```python
from build123d import *

# Parameters (mm, degrees)
SKETCH2_R              = 14.2875
SKETCH2_W              = 81.28
SKETCH2_H              = 3.175
BOSS_EXTRUDE1_DEPTH    = 3.175
SKETCH9_R              = 14.2875
CUT_EXTRUDE2_DEPTH     = 3.175
SKETCH2_3_W            = 81.28
SKETCH2_3_H            = 3.175
BOSS_EXTRUDE2_DEPTH    = 60.7695
BOSS_EXTRUDE3_DEPTH    = 3.175
FILLET1_R              = 2.54
FILLET2_R              = 42.2275
CONVERT_SOLID2_START   = -102
CONVERT_SOLID2_DEPTH   = 184
CONVERT_SOLID2_2_DEPTH = 81.28
UNFOLD1_START          = -51
UNFOLD1_DEPTH          = 132.28
UNFOLD1_2_DEPTH        = 78.74
UNFOLD1_START_2        = 0.13716
UNFOLD1_3_DEPTH        = 3.03784
FOLD1_START            = -58.892012294
FOLD1_OUTLINE_W        = 3.03784
FOLD1_OUTLINE_H        = 81.28
FOLD1_DEPTH            = 59.530319476
FOLD1_2_DEPTH          = 6.21284
FOLD1_START_2          = -49.557397552
FOLD1_3_DEPTH          = 131.557397552


with BuildPart() as part:
    # Sketch2 → Boss-Extrude1 (new body)
    # profile 1 of 2: a face of its own
    with BuildSketch(Plane(origin=(0, 0, 0), x_dir=(0, 0, -1), z_dir=(1, 0, 0))):
        with BuildLine():
            Line((0, 3.175), (0, 69.85))
            Line((0, 69.85), (89.183866464, 160.063269699))
            ThreePointArc((89.183866464, 160.063269699), (97.582743975, 203.257963311), (60.96, 227.65258))
            Line((60.96, 227.65258), (-81.28, 227.65258))
            Line((-81.28, 227.65258), (-81.28, 69.85))
            Line((-81.28, 69.85), (-81.28, 3.175))
            Line((-81.28, 3.175), (0, 3.175))
        make_face()
        with Locations((60.96, 187.96508)):
            Circle(SKETCH2_R, mode=Mode.SUBTRACT)
    # profile 2 of 2: a face of its own
    with BuildSketch(Plane(origin=(0, 0, 0), x_dir=(0, 0, -1), z_dir=(1, 0, 0))):
        with Locations((-40.64, 1.5875)):
            Rectangle(SKETCH2_W, SKETCH2_H)
    extrude(amount=BOSS_EXTRUDE1_DEPTH)

    # Sketch9 → Cut-Extrude2 (cut)
    with BuildSketch(Plane(origin=(0, 0, 0), x_dir=(0, 0, -1), z_dir=(1, 0, 0))):
        with Locations((-49.5046, 74.46228868)):
            Circle(SKETCH9_R)
    extrude(amount=CUT_EXTRUDE2_DEPTH, mode=Mode.SUBTRACT)

    # Sketch2<3> → Boss-Extrude2 (add)
    with BuildSketch(Plane(origin=(0, 0, 0), x_dir=(0, 0, -1), z_dir=(1, 0, 0))):
        with Locations((-40.64, 1.5875)):
            Rectangle(SKETCH2_3_W, SKETCH2_3_H)
    extrude(amount=-BOSS_EXTRUDE2_DEPTH)

    # Sketch3 → Boss-Extrude3 (add)
    with BuildSketch(Plane(origin=(0, 3.175, 0), x_dir=(1, 0, 0), z_dir=(0, 1, 0))):
        Polygon((-60.7695, 0), (-60.7695, 53.1495), (-7.62, 0), align=None)
    extrude(amount=-BOSS_EXTRUDE3_DEPTH)

    # Fillet1
    fillet1_edges = [part.edges().sort_by_distance(p)[0] for p in [
        (-60.7695, 1.5875, 81.28),
        (-60.7695, 1.5875, -53.1495),
    ]]
    fillet(fillet1_edges, radius=FILLET1_R)

    # Fillet2
    fillet2_edges = [part.edges().sort_by_distance(p)[0] for p in [
        (1.5875, 227.65258, 81.28),
    ]]
    fillet(fillet2_edges, radius=FILLET2_R)

    # Convert-Solid2: read off the stored shape, not the designer's step
    # Convert-Solid2 outline → Convert-Solid2 (cut)
    with BuildSketch(Plane.XY.offset(CONVERT_SOLID2_START)):
        with BuildLine():
            ThreePointArc((3.175, 6.21284), (1.355301294, 1.819698706), (-3.03784, 0))
            Line((-3.03784, 0), (3.175, 0))
            Line((3.175, 0), (3.175, 6.21284))
        make_face()
        with BuildLine():
            Line((-60.7695, 3.175), (-60.7695, 3.03784))
            Line((-60.7695, 3.03784), (-3.03784, 3.03784))
            ThreePointArc((-3.03784, 3.03784), (-2.571212204, 3.072317193), (-2.114718593, 3.175))
            Line((-2.114718593, 3.175), (-60.7695, 3.175))
        make_face()
        with BuildLine():
            Line((0.13716, 6.21284), (0.13716, 227.65258))
            Line((0.13716, 227.65258), (0, 227.65258))
            Line((0, 227.65258), (0, 5.289718593))
            ThreePointArc((0, 5.289718593), (0.102682807, 5.746212204), (0.13716, 6.21284))
        make_face()
    extrude(amount=CONVERT_SOLID2_DEPTH, mode=Mode.SUBTRACT)

    # Convert-Solid2 2 outline → Convert-Solid2 2 (add)
    with BuildSketch(Plane.XY):
        with BuildLine():
            ThreePointArc((0, 5.289718593), (-0.79277597, 3.96777597), (-2.114718593, 3.175))
            Line((-2.114718593, 3.175), (0, 3.175))
            Line((0, 3.175), (0, 5.289718593))
        make_face()
    extrude(amount=CONVERT_SOLID2_2_DEPTH)

    # Unfold1: read off the stored shape, not the designer's step
    # Unfold1 outline → Unfold1 (cut)
    with BuildSketch(Plane.XY.offset(UNFOLD1_START)):
        with BuildLine():
            ThreePointArc((-3.03784, 0), (-1.391483498, 0.222106228), (0.13716, 0.872544516))
            Line((0.13716, 0.872544516), (0.13716, 6.21284))
            ThreePointArc((0.13716, 6.21284), (-0.79277597, 3.96777597), (-3.03784, 3.03784))
            Line((-3.03784, 3.03784), (-60.7695, 3.03784))
            Line((-60.7695, 3.03784), (-60.7695, 0))
            Line((-60.7695, 0), (-3.03784, 0))
        make_face()
    extrude(amount=UNFOLD1_DEPTH, mode=Mode.SUBTRACT)

    # Unfold1 2 outline → Unfold1 2 (add)
    with BuildSketch(Plane.XY):
        with BuildLine():
            Line((0.13716, -58.892012294), (3.175, -58.892012294))
            Line((3.175, -58.892012294), (3.175, 6.21284))
            ThreePointArc((3.175, 6.21284), (2.362398322, 3.140901373), (0.13716, 0.872544516))
            Line((0.13716, 0.872544516), (0.13716, -58.892012294))
        make_face()
    extrude(amount=UNFOLD1_2_DEPTH)

    # Unfold1 3 outline → Unfold1 3 (add)
    with BuildSketch(Plane.YZ.offset(UNFOLD1_START_2)):
        with BuildLine():
            Line((8, 81.28), (-56.352012294, 81.28))
            ThreePointArc((-56.352012294, 81.28), (-58.148063518, 80.536051224), (-58.892012294, 78.74))
            Line((-58.892012294, 78.74), (8, 78.74))
            Line((8, 78.74), (8, 81.28))
        make_face()
        with BuildLine():
            Line((-5.742512294, 0), (-58.892012294, 0))
            Line((-58.892012294, 0), (-58.892012294, -47.017397552))
            ThreePointArc((-58.892012294, -47.017397552), (-57.324028212, -49.364051564), (-54.55596107, -48.813448776))
            Line((-54.55596107, -48.813448776), (-5.742512294, 0))
        make_face()
    extrude(amount=UNFOLD1_3_DEPTH)

    # Fold1: read off the stored shape, not the designer's step
    # Fold1 outline → Fold1 (cut)
    with BuildSketch(Plane(origin=(0, 0, 0), x_dir=(1, 0, 0), z_dir=(0, 1, 0)).offset(FOLD1_START)):
        with Locations((1.65608, -40.64)):
            Rectangle(FOLD1_OUTLINE_W, FOLD1_OUTLINE_H)
    extrude(amount=FOLD1_DEPTH, mode=Mode.SUBTRACT)

    # Fold1 2 outline → Fold1 2 (add)
    with BuildSketch(Plane(origin=(0, 0, 0), x_dir=(1, 0, 0), z_dir=(0, 1, 0))):
        with BuildLine():
            ThreePointArc((-60.7695, -78.74), (-60.025551224, -80.536051224), (-58.2295, -81.28))
            Line((-58.2295, -81.28), (0.13716, -81.28))
            Line((0.13716, -81.28), (0.13716, 0))
            Line((0.13716, 0), (-7.62, 0))
            Line((-7.62, 0), (-56.433448776, 48.813448776))
            ThreePointArc((-56.433448776, 48.813448776), (-59.201515918, 49.364051564), (-60.7695, 47.017397552))
            Line((-60.7695, 47.017397552), (-60.7695, -78.74))
        make_face()
    extrude(amount=FOLD1_2_DEPTH)

    # Fold1 3 outline → Fold1 3 (cut)
    with BuildSketch(Plane.XY.offset(FOLD1_START_2)):
        with BuildLine():
            Line((-60.7695, 6.21284), (-60.7695, 3.03784))
            Line((-60.7695, 3.03784), (-3.03784, 3.03784))
            ThreePointArc((-3.03784, 3.03784), (-0.79277597, 3.96777597), (0.13716, 6.21284))
            Line((0.13716, 6.21284), (-60.7695, 6.21284))
        make_face()
        with BuildLine():
            Line((-3.03784, 0), (-60.7695, -1.4e-08))
            Line((-60.7695, -1.4e-08), (-60.7695, -60))
            Line((-60.7695, -60), (0.13716, -60))
            Line((0.13716, -60), (0.13716, -58.892012294))
            Line((0.13716, -58.892012294), (3.175, -58.892012294))
            Line((3.175, -58.892012294), (3.175, 6.21284))
            ThreePointArc((3.175, 6.21284), (1.355301294, 1.819698706), (-3.03784, 0))
        make_face()
    extrude(amount=FOLD1_3_DEPTH, mode=Mode.SUBTRACT)


solid = part.part
```
Here's how the part is built. I have some questions about the finished solid (model axes, mm). A direction names the side the tool comes from. Give positions to 0.01 mm unless a question says otherwise; leave off trailing zeros. Write each loop counter-clockwise with the first axis right and the second up, starting at its lowest first coordinate (ties: lowest second). Pieces come first, ordered by that corner, then holes. Notation, with made-up numbers: (36.5, 61) -> (58.5, 61) arc R23 cw to (58.5, 77) -> close; hole circle Ø7 at (58, 49). An arc over 180 degrees is marked (long way). Write each question's results on one line, items separated by ' | '.
Item 1: Suppose I cut it at B-B on y = 179.5. Write out the boundary of the cut face in (x, z) (3 decimals), plus the area to 3 significant figures.
Output:
outline: (0.137, -99.734) -> (3.175, -99.734) -> (3.175, -72.47) -> (0.137, -72.47) -> close; (0.137, -49.45) -> (3.175, -49.45) -> (3.175, 81.28) -> (0.137, 81.28) -> close | area: 480 mm^2
Item 2: Suppose I cut it at D-D on x = -16.5. Write out the boundary of the cut face in (y, z), plus the area to 3 significant figures.
Output:
outline: (0, -8.88) -> (3.04, -8.88) -> (3.04, 81.28) -> (0, 81.28) -> close | area: 274 mm^2
Item 3: For pin 1 Ø6 at (x, z) = (-37, 49) entering from +Y; pin 2 Ø2 at (y, z) = (110, -3) entering from -X, each with a flat end and sliding along its axis, tell me the tip position at first contact or that it passes through.
Output:
pin 1: stops at y = 3.04 | pin 2: stops at x = 0.14
Item 4: If I drill on L1, parallel to Y at x = -16, z = 20; L2, parallel to X at y = 194, z = -7 (3 decimals), over which ranges is the centre line in solid material (lowest first)?
Output:
L1: y = 0 to 3.04 | L2: x = 0.137 to 3.175
Item 5: Suppose I cut it at C-C on z = -20. Write out the boundary of the cut face in (x, y) (1 decimal).
Output:
outline: (-60.8, 0) -> (-27.6, 0) -> (-27.6, 3) -> (-60.8, 3) -> close; (0.1, 90.1) -> (3.2, 90.1) -> (3.2, 227.7) -> (0.1, 227.7) -> close
Item 6: On a 3-axis mill with a long thin cutter (end or side, diameter ignored), from which of +Z, -Z, +X, -X, +Y, -Y can I reach the whole of each face in a straight line? I mean faces 5 (the face through (0.137, 143, 9)), 6 (the face through (1.403, 1.868, 40.071)). Say none if no direction works.
Output:
face 5: +Z, -Z, -X, +Y | face 6: +Z, -Z, +X, -Y
Item 7: We'd pull the mould along Y, two halves only. Please class faces 1 (the face through (1.6, 179.3, -49.6)), 2 (the face through (-32, 3.038, 29)), 3 (the face through (1.63, 114.33, -43.97)), 4 (the face through (-31.69, 1.5, -24.07)): pulls with the +Y half, pulls with the -Y half, needs draft (parallel to the pull), parting line crosses it, or undercut.
Output:
face 1: undercut | face 2: pulls with the +Y half | face 3: pulls with the -Y half | face 4: needs draft
